Check sheet for the modelled part. Datum: model origin and axes. Units: mm. Give positions to 0.01 mm unless a question says otherwise; leave off trailing zeros. Loops run counter-clockwise (first coordinate to the right, second up) from the corner with the lowest first, then second, coordinate; pieces in that order, holes last. Notation, with made-up numbers: M 49.25,54 L 56.25,54 A10 ccw 56.25,66 Z; hole C 6,-26.5 d7. An arc over 180 degrees is marked long. Put each result on its own line as item: value. Start each with the question number.
```python
from build123d import *

# Parameters (mm, degrees)
SKETCH1_R           = 340
SKETCH1_R_2         = 250
BOSS_EXTRUDE1_DEPTH = 10
BOSS_EXTRUDE2_DEPTH = 10
FILLET1_R           = 10


with BuildPart() as part:
    # Sketch1 → Boss-Extrude1 (new body)
    with BuildSketch(Plane(origin=(0, 0, 0), x_dir=(1, 0, 0), z_dir=(0, 1, 0))):
        Circle(SKETCH1_R)
        Circle(SKETCH1_R_2, mode=Mode.SUBTRACT)
    extrude(amount=BOSS_EXTRUDE1_DEPTH)

    # Sketch2 → Boss-Extrude2 (add)
    with BuildSketch(Plane.XZ):
        with BuildLine():
            Line((371.651718683, -60), (334.664010614, -60))
            ThreePointArc((334.664010614, -60), (340, 0), (334.664010614, 60))
            Line((334.664010614, 60), (371.651718683, 60))
            ThreePointArc((371.651718683, 60), (378.234524569, 57.527726527), (381.562431181, 51.333333333))
            ThreePointArc((381.562431181, 51.333333333), (385, 0), (381.562431181, -51.333333333))
            ThreePointArc((381.562431181, -51.333333333), (378.234524569, -57.527726527), (371.651718683, -60))
        make_face()
        with BuildLine():
            ThreePointArc((363.611064803, 31.811846103), (365, 0), (363.611064803, -31.811846103))
            ThreePointArc((363.611064803, -31.811846103), (358.194312599, -36.35704088), (353.649117823, -30.940288675))
            ThreePointArc((353.649117823, -30.940288675), (355, 0), (353.649117823, 30.940288675))
            ThreePointArc((353.649117823, 30.940288675), (358.194312599, 36.35704088), (363.611064803, 31.811846103))
        make_face(mode=Mode.SUBTRACT)
        with BuildLine():
            Line((-133.864335114, 351.85982974), (-115.37048108, 319.827534924))
            ThreePointArc((-115.37048108, 319.827534924), (-170, 294.448637287), (-219.293529534, 259.827534924))
            Line((-219.293529534, 259.827534924), (-237.787383569, 291.85982974))
            ThreePointArc((-237.787383569, 291.85982974), (-238.937734879, 298.796843602), (-235.237186318, 304.776091866))
            ThreePointArc((-235.237186318, 304.776091866), (-192.5, 333.419780457), (-146.325244863, 356.109425199))
            ThreePointArc((-146.325244863, 356.109425199), (-139.29678969, 356.324570129), (-133.864335114, 351.85982974))
        make_face()
        with BuildLine():
            ThreePointArc((-209.355399268, 298.990496165), (-210.583277308, 292.026853762), (-203.619634905, 290.798975723))
            ThreePointArc((-203.619634905, 290.798975723), (-177.5, 307.439018343), (-150.029482918, 321.739264398))
            ThreePointArc((-150.029482918, 321.739264398), (-147.611035291, 328.383894642), (-154.255665535, 330.802342268))
            ThreePointArc((-154.255665535, 330.802342268), (-182.5, 316.099272381), (-209.355399268, 298.990496165))
        make_face(mode=Mode.SUBTRACT)
        with BuildLine():
            Line((-237.787383569, -291.85982974), (-219.293529534, -259.827534924))
            ThreePointArc((-219.293529534, -259.827534924), (-170, -294.448637287), (-115.37048108, -319.827534924))
            Line((-115.37048108, -319.827534924), (-133.864335114, -351.85982974))
            ThreePointArc((-133.864335114, -351.85982974), (-139.29678969, -356.324570129), (-146.325244863, -356.109425199))
            ThreePointArc((-146.325244863, -356.109425199), (-192.5, -333.419780457), (-235.237186318, -304.776091866))
            ThreePointArc((-235.237186318, -304.776091866), (-238.937734879, -298.796843602), (-237.787383569, -291.85982974))
        make_face()
        with BuildLine():
            ThreePointArc((-154.255665535, -330.802342268), (-182.5, -316.099272381), (-209.355399268, -298.990496165))
            ThreePointArc((-209.355399268, -298.990496165), (-210.583277308, -292.026853762), (-203.619634905, -290.798975723))
            ThreePointArc((-203.619634905, -290.798975723), (-177.5, -307.439018343), (-150.029482918, -321.739264398))
            ThreePointArc((-150.029482918, -321.739264398), (-147.611035291, -328.383894642), (-154.255665535, -330.802342268))
        make_face(mode=Mode.SUBTRACT)
    extrude(amount=-BOSS_EXTRUDE2_DEPTH)

    # Fillet1
    fillet1_edges = [part.edges().sort_by_distance(p)[0] for p in [
        (334.664010614, 5, -60),
        (334.664010614, 5, 60),
        (-115.37048108, 5, 319.827534924),
        (-219.293529534, 5, 259.827534924),
        (-219.293529534, 5, -259.827534924),
        (-115.37048108, 5, -319.827534924),
    ]]
    fillet(fillet1_edges, radius=FILLET1_R)


solid = part.part
```
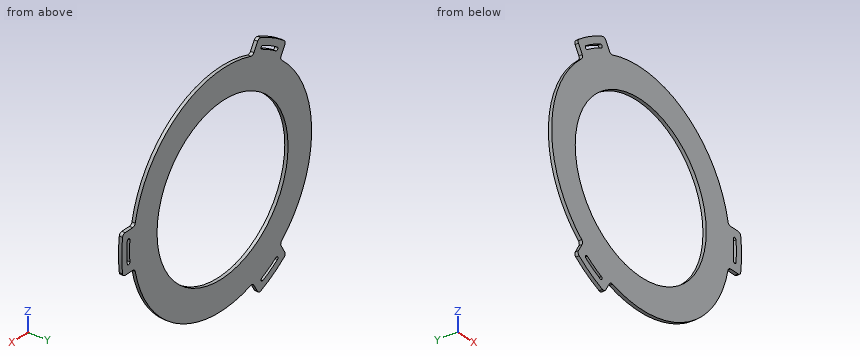
Q1. Thickness scan on line 1 along Z through (x, y) = (0, 6); line 2 along X through (y, z) = (5, -217.5); line 3 along X through (y, z) = (9.5, 69). Record the ranges inside material, lowest first. Write a range as [from, to].
Q2. Section check A-A, the plane z = 0. Record the cut outline in (x, y).
Q3. Section check D-D, the plane y = 6.5. Give the number of separate pieces and of enclosed holes in the cut face, then the cut area to 3 significant figures.
Q4. Section check C-C, the plane x = 95. Record the cut outline in (y, z).
Q5. Depth check by flat-ended pin: P1, Ø1.5, axis at x = -215.5, y = 2, coming from the +Z side; P2, Ø3, axis at y = 5.5, z = 75, coming from the -X side; P3, Ø5, axis at x = 357.5, y = 4, coming from the -Z side. Enter the tip coordinate at first touch or a pass-through.
Q6. Section check B-B, the plane x = 0. Record the cut outline in (y, z).
Found:
1. line 1: z = [-340, -250], [250, 340]
1. line 2: x = [-261.33, -123.26], [123.26, 261.33]
1. line 3: x = [-332.92, -240.29], [240.29, 332.92]
2. outline: M -340,0 L -250,0 L -250,10 L -340,10 Z; M 250,0 L 355,0 L 355,10 L 250,10 Z; M 365,0 L 385,0 L 385,10 L 365,10 Z
3. separate pieces: 1
3. enclosed holes: 4
3. area: 181,000 mm^2
4. outline: M 0,-326.46 L 10,-326.46 L 10,-231.25 L 0,-231.25 Z; M 0,231.25 L 10,231.25 L 10,326.46 L 0,326.46 Z
5. P1: stops at z = 319.54
5. P2: stops at x = -331.96
5. P3: stops at z = -60
6. outline: M 0,-340 L 10,-340 L 10,-250 L 0,-250 Z; M 0,250 L 10,250 L 10,340 L 0,340 Z
